```python
from build123d import *

# Parameters (mm, degrees)
SKETCH_1_W          = 20
SKETCH_1_H          = 30
SKETCH_1_R          = 1.5
EXTRUDE_1_DEPTH     = 4
SKETCH_2_W          = 30
SKETCH_2_H          = 4
EXTRUDE_2_DEPTH     = 24
FILLET_1_R          = 3
SKETCH_3_R          = 8
CUT_EXTRUDE_1_DEPTH = 24
FILLET_2_R          = 3
FILLET_3_R          = 4
FILLET_4_R          = 4


with BuildPart() as part:
    # 草图1 → 凸台-拉伸1 (new body)
    with BuildSketch(Plane.XY):
        Rectangle(SKETCH_1_W, SKETCH_1_H)
        with Locations((-5, 3)):
            Circle(SKETCH_1_R, mode=Mode.SUBTRACT)
        with Locations((5, 3)):
            Circle(SKETCH_1_R, mode=Mode.SUBTRACT)
        with Locations((-5, -7)):
            Circle(SKETCH_1_R, mode=Mode.SUBTRACT)
        with Locations((5, -7)):
            Circle(SKETCH_1_R, mode=Mode.SUBTRACT)
    extrude(amount=EXTRUDE_1_DEPTH)

    # 草图2 → 凸台-拉伸2 (add)
    with BuildSketch(Plane(origin=(0, 15, 0), x_dir=(1, 0, 0), z_dir=(0, 1, 0))):
        with Locations((0, -2)):
            Rectangle(SKETCH_2_W, SKETCH_2_H)
    extrude(amount=EXTRUDE_2_DEPTH)

    # 圆角1
    fillet_1_edges = [part.edges().sort_by_distance(p)[0] for p in [
        (-10, 15, 2),
        (10, 15, 2),
    ]]
    fillet(fillet_1_edges, radius=FILLET_1_R)

    # 草图3 → 切除-拉伸1 (cut)
    with BuildSketch(Plane.XY.offset(4)):
        with Locations((0, 26.5)):
            Circle(SKETCH_3_R)
    extrude(amount=-CUT_EXTRUDE_1_DEPTH, mode=Mode.SUBTRACT)

    # 圆角2
    fillet_2_edges = [part.edges().sort_by_distance(p)[0] for p in [
        (15, 15, 2),
        (15, 39, 2),
        (-15, 39, 2),
        (-15, 15, 2),
    ]]
    fillet(fillet_2_edges, radius=FILLET_2_R)

    # 圆角3
    fillet_3_edges = [part.edges().sort_by_distance(p)[0] for p in [
        (-10, -15, 2),
    ]]
    fillet(fillet_3_edges, radius=FILLET_3_R)

    # 圆角4
    fillet_4_edges = [part.edges().sort_by_distance(p)[0] for p in [
        (10, -15, 2),
    ]]
    fillet(fillet_4_edges, radius=FILLET_4_R)


solid = part.part
```
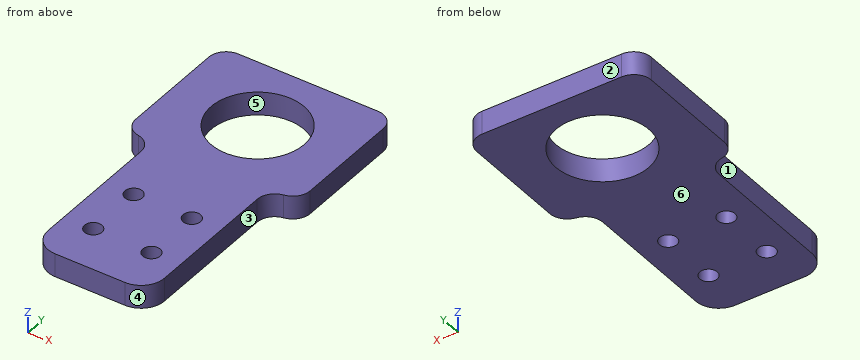
Part model, mm, in its own coordinate system. Face numbers are marked on the shaded views. A direction names the side the tool comes from. Round coordinates to 2 decimals unless told otherwise and drop trailing zeros. Loops run counter-clockwise (first coordinate to the right, second up) from the corner with the lowest first, then second, coordinate; pieces in that order, holes last.
1. Slice it at B-B (x = 0). Give the cut face in (y, z), and give its area (3 significant figures).
Solutions:
outline: (-15, 0) - (18.5, 0) - (18.5, 4) - (-15, 4) - close; (34.5, 0) - (39, 0) - (39, 4) - (34.5, 4) - close
area: 152 mm2
2. Slice it at D-D (x = 5.5). Give the cut face in (y, z).
Solutions:
outline: (-15, 0) - (-8.41, 0) - (-8.41, 4) - (-15, 4) - close; (-5.59, 0) - (1.59, 0) - (1.59, 4) - (-5.59, 4) - close; (4.41, 0) - (20.69, 0) - (20.69, 4) - (4.41, 4) - close; (32.31, 0) - (39, 0) - (39, 4) - (32.31, 4) - close
3. Two-plate mould, pull along X, no slides. Class the marked faces 4, 5 and 6: pulls with the +X half, pulls with the -X half, needs draft (parallel to the pull), parting line crosses it, or undercut.
Solutions:
face 4: pulls with the +X half
face 5: undercut
face 6: needs draft
4. Slice it at C-C (y = 3). Give the cut face in (x, z).
Solutions:
outline: (-10, 0) - (-6.5, 0) - (-6.5, 4) - (-10, 4) - close; (-3.5, 0) - (3.5, 0) - (3.5, 4) - (-3.5, 4) - close; (6.5, 0) - (10, 0) - (10, 4) - (6.5, 4) - close
5. 3-axis set-ups, long thin cutter, end or side, ignore diameter. For the marked faces 1, 2 and 3: which of +Z, -Z, +X, -X, +Y, -Y reach the whole face in a straight line?
Solutions:
face 1: +Z, -Z, -X, -Y
face 2: +Z, -Z, +X, -X, +Y
face 3: +Z, -Z, +X, -Y
6. Slice it at A-A (y = 26.5). Give the cut face in (x, z).
Solutions:
outline: (-15, 0) - (-8, 0) - (-8, 4) - (-15, 4) - close; (8, 0) - (15, 0) - (15, 4) - (8, 4) - close
7. Drill centre lines: line 1 along Y through (x, z) = (0, 1.3); line 2 along Y through (x, z) = (5, 1.8) (3 decimals); line 3 along Y through (x, z) = (2, 0.4). Where is each one in solid material? Low to high.
Solutions:
line 1: y = -15 to 18.5, 34.5 to 39
line 2: y = -15 to -8.5, -5.5 to 1.5, 4.5 to 20.255, 32.745 to 39
line 3: y = -15 to 18.75, 34.25 to 39
8. Flat gauge pins, fed straight in: pin 1 (4 mm diameter, centred on x = 2.5, y = 19.5, fed in from +Z); pin 2 (2.5 mm diameter, centred on x = -5, y = -7, fed in from +Z). Where does each tip first touch, or does it go through?
Solutions:
pin 1: stops at z = 4
pin 2: passes through
